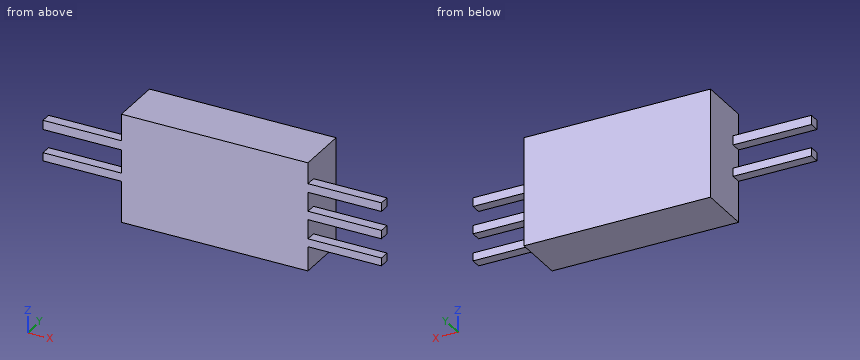
from build123d import *

# Parameters (mm, degrees)
SKETCH1_W           = 67
SKETCH1_H           = 39
BOSS_EXTRUDE1_DEPTH = 18.7
SKETCH2_W           = 28.153869909
SKETCH2_H           = 3.308256434
SKETCH2_H_2         = 2.957380752
SKETCH2_W_2         = 26.399491497
SKETCH2_H_3         = 3.107756044
SKETCH2_H_4         = 3.018867182
SKETCH2_H_5         = 2.841286759
BOSS_EXTRUDE2_DEPTH = 3.7


with BuildPart() as part:
    # Sketch1 → Boss-Extrude1 (new body)
    with BuildSketch(Plane(origin=(0, 0, 0), x_dir=(1, 0, 0), z_dir=(0, 1, 0))):
        with Locations((33.5, 19.5)):
            Rectangle(SKETCH1_W, SKETCH1_H)
    extrude(amount=BOSS_EXTRUDE1_DEPTH)

    # Sketch2 → Boss-Extrude2 (add)
    with BuildSketch(Plane.XZ):
        with Locations((-14.076934955, -11.229358915)):
            Rectangle(SKETCH2_W, SKETCH2_H)
        with Locations((-14.076934955, -22.733068788)):
            Rectangle(SKETCH2_W, SKETCH2_H_2)
        with Locations((80.199745748, -9.073979723)):
            Rectangle(SKETCH2_W_2, SKETCH2_H_3)
        with Locations((80.199745748, -18.984327025)):
            Rectangle(SKETCH2_W_2, SKETCH2_H_4)
        with Locations((80.199745748, -28.84004047)):
            Rectangle(SKETCH2_W_2, SKETCH2_H_5)
    extrude(amount=-BOSS_EXTRUDE2_DEPTH)


solid = part.part
Check sheet for the modelled part. Datum: model origin and axes. Units: mm. Give positions to 0.01 mm unless a question says otherwise; leave off trailing zeros. Loops run counter-clockwise (first coordinate to the right, second up) from the corner with the lowest first, then second, coordinate; pieces in that order, holes last. Notation, with made-up numbers: M -30,-23.5 L -17,-23.5 A18 ccw -17,-8.5 Z; hole C 80.5,34 d11. An arc over 180 degrees is marked long. Use a Markdown table: item, result. Add a question column.
Q1. Sectioned sample at D-D, the plane z = -29. Record the cut outline in (x, y), then the cut area to 3 significant figures.
Q2. Scan line: line 1 along X through (y, z) = (1, -14.5). Record every from-to range of solid material in increasing order. Write a range as [from, to].
Q3. Sectioned sample at C-C, the plane x = 72. Record the cut outline in (y, z), then the cut area to 3 significant figures.
Q4. Sectioned sample at B-B, the plane y = 2. Record the cut outline in (x, z).
Q5. Go/stop test with flat-tipped pins: pin 1 (4 mm diameter, centred on x = 74, y = 1.5, fed in from -Z); pin 2 (6 mm diameter, centred on y = 5, z = -16.5, fed in from -X); pin 3 (1.7 mm diameter, centred on x = -17.5, z = -12, fed in from +Y); pin 4 (6 mm diameter, centred on x = -8, y = 8.5, fed in from +Z). Record where each tip stops, or that it passes through.
Q6. Sectioned sample at A-A, the plane x = -15.5. Record the cut outline in (y, z).
Verdict:
| question | item | result |
|---|---|---|
| 1 | outline | M 0,0 L 93.4,0 L 93.4,3.7 L 67,3.7 L 67,18.7 L 0,18.7 Z |
| 1 | area | 1,350 mm^2 |
| 2 | line 1 | [0, 67] |
| 3 | outline | M 0,-30.26 L 3.7,-30.26 L 3.7,-27.42 L 0,-27.42 Z; M 0,-20.49 L 3.7,-20.49 L 3.7,-17.47 L 0,-17.47 Z; M 0,-10.63 L 3.7,-10.63 L 3.7,-7.52 L 0,-7.52 Z |
| 3 | area | 33.2 mm^2 |
| 4 | outline | M -28.15,-24.21 L 0,-24.21 L 0,-39 L 67,-39 L 67,-30.26 L 93.4,-30.26 L 93.4,-27.42 L 67,-27.42 L 67,-20.49 L 93.4,-20.49 L 93.4,-17.47 L 67,-17.47 L 67,-10.63 L 93.4,-10.63 L 93.4,-7.52 L 67,-7.52 L 67,0 L 0,0 L 0,-9.58 L -28.15,-9.58 L -28.15,-12.88 L 0,-12.88 L 0,-21.25 L -28.15,-21.25 Z |
| 5 | pin 1 | z = -30.26 |
| 5 | pin 2 | x = 0 |
| 5 | pin 3 | y = 3.7 |
| 5 | pin 4 | through |
| 6 | outline | M 0,-24.21 L 3.7,-24.21 L 3.7,-21.25 L 0,-21.25 Z; M 0,-12.88 L 3.7,-12.88 L 3.7,-9.58 L 0,-9.58 Z |
